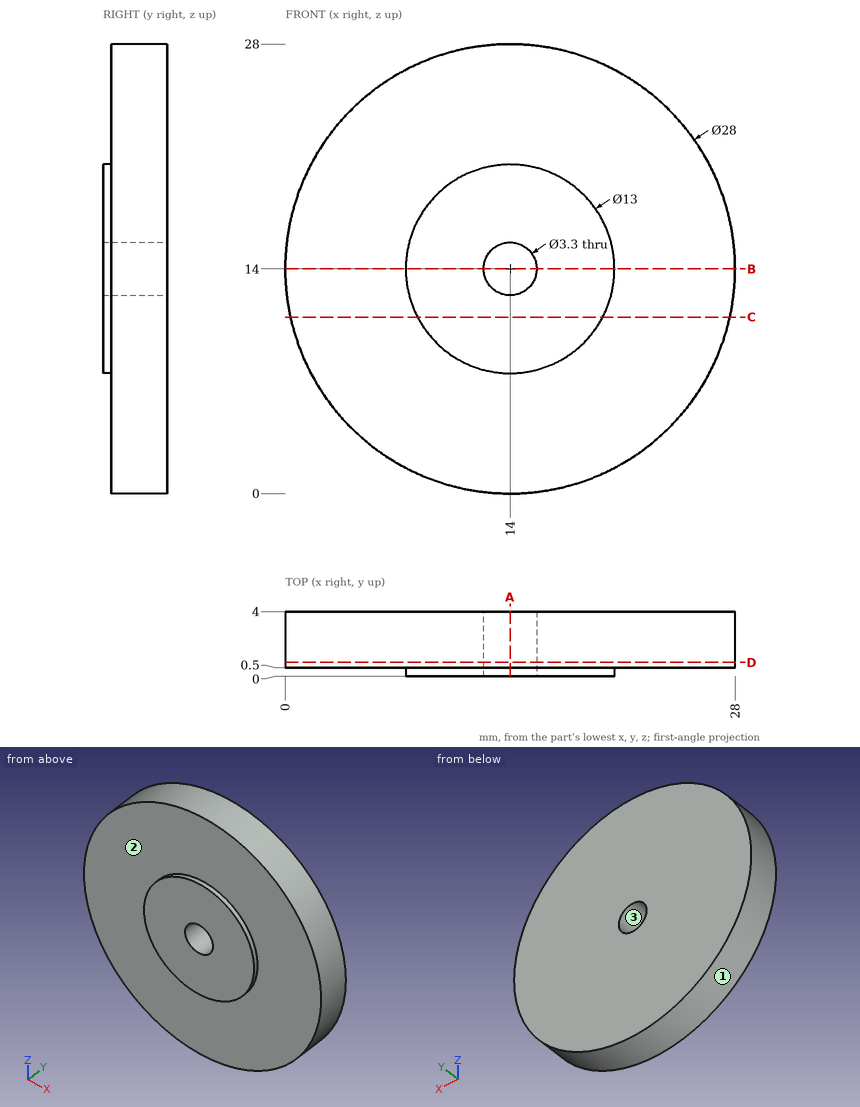
Job drawing, mm, ordinate dimensions from the low corner. One solid piece. Coordinates: 2 decimals unless noted, no trailing zeros. Write each loop counter-clockwise with the first axis right and the second up, starting at its lowest first coordinate (ties: lowest second). Pieces come first, ordered by that corner, then holes.
Item 1: Mould opens along X. For the marked faces 1, 2 and 3 say: released by +X, released by -X, zero draft, split by the parting line, or undercut.
Item 2: Pin check, flat tips, straight feed: pin 1 (1.5 mm diameter, centred on x = 24.5, y = 1.5, fed in from -Z); pin 2 (4 mm diameter, centred on x = 14, z = 14, fed in from -Y); pin 3 (1.5 mm diameter, centred on y = 0.5, z = 19.5, fed in from -X). Stop position of each tip, or through.
Item 3: Slice it at D-D (y = 0.85). Write the cut outline in (x, z).
Item 4: Probe line 1 (Z direction, x = 14, y = 2.05); line 2 (Y direction, x = 8.5, z = 19.5). List the from-to ranges inside material, lowest first.
Item 5: Slice it at C-C (z = 11). Write the cut outline in (x, y), and give its area (3 significant figures).
Item 6: Slice it at A-A (x = 14). Write the cut outline in (y, z).
Item 7: Slice it at B-B (z = 14). Write the cut outline in (x, y), and give its area (3 significant figures).
Results found:
1. face 1: split by the parting line
1. face 2: zero draft
1. face 3: undercut
2. pin 1: stops at z = 3.95
2. pin 2: stops at y = 0
2. pin 3: stops at x = 0.83
3. outline: circle Ø28 at (14, 14); hole circle Ø3.3 at (14, 14)
4. line 1: z = 0 to 12.35, 15.65 to 28
4. line 2: y = 0.5 to 4
5. outline: (0.33, 0.5) - (8.23, 0.5) - (8.23, 0) - (19.77, 0) - (19.77, 0.5) - (27.67, 0.5) - (27.67, 4) - (0.33, 4) - close
5. area: 101 mm2
6. outline: (0, 7.5) - (0.5, 7.5) - (0.5, 0) - (4, 0) - (4, 12.35) - (0, 12.35) - close; (0, 15.65) - (4, 15.65) - (4, 28) - (0.5, 28) - (0.5, 20.5) - (0, 20.5) - close
7. outline: (0, 0.5) - (7.5, 0.5) - (7.5, 0) - (12.35, 0) - (12.35, 4) - (0, 4) - close; (15.65, 0) - (20.5, 0) - (20.5, 0.5) - (28, 0.5) - (28, 4) - (15.65, 4) - close
7. area: 91.3 mm2
